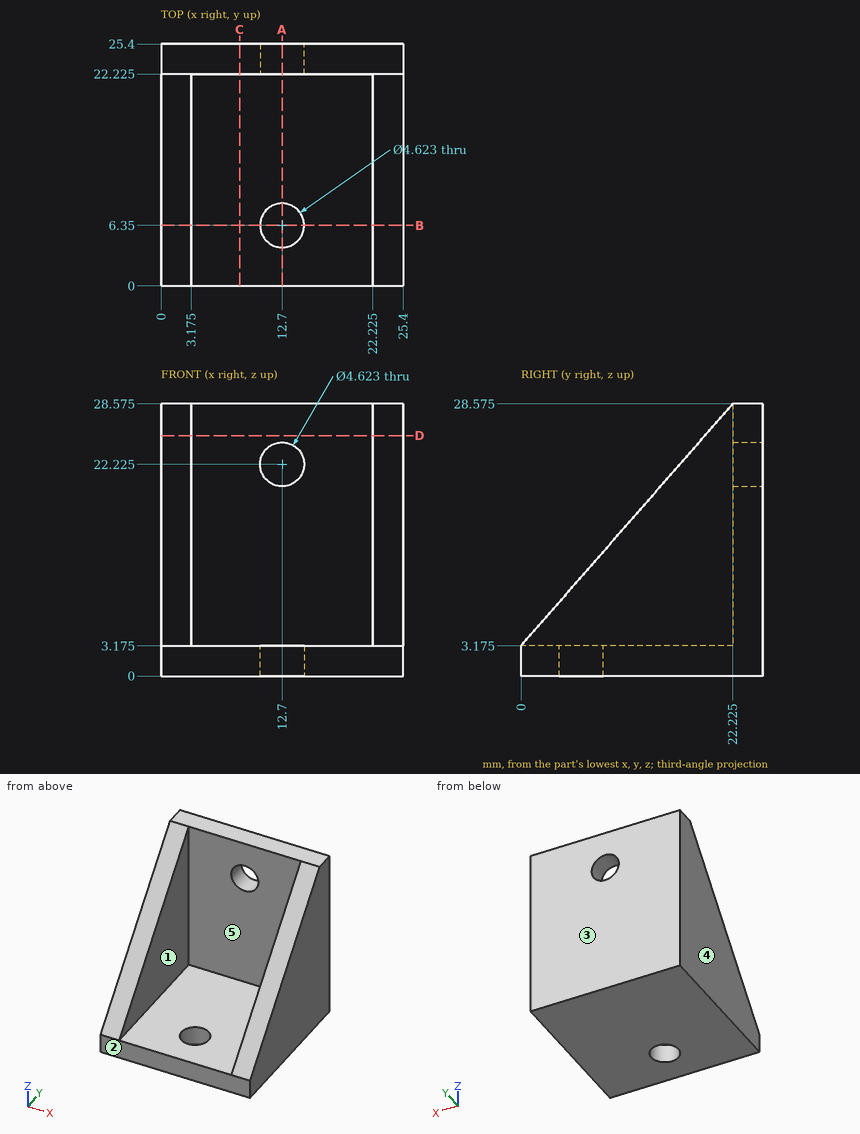
Source: three-view drawing plus pictorial views. Frame: mm from the lowest corner of the part. A direction names the side the tool comes from. Round coordinates to 2 decimals unless told otherwise and drop trailing zeros. Loops run counter-clockwise (first coordinate to the right, second up) from the corner with the lowest first, then second, coordinate; pieces in that order, holes last.
1. Section query A-A on x = 12.7. Output: boundary loops of the cut face in (y, z) (1 decimal).
2. Section query B-B on y = 6.35. Output: boundary loops of the cut face in (x, z) (1 decimal), and give its area (3 significant figures).
3. Section query D-D on z = 25.25. Output: boundary loops of the cut face in (x, y) (1 decimal).
4. Ray query, L1, parallel to X at y = 16.5, z = 11.5 (3 decimals); L2, parallel to Y at x = 12.7, z = 2.4; L3, parallel to Z at x = 12.7, y = 22.9 (1 decimal). Return the intervals inside material, ascending.
5. Contact query for flat-ended pins moving along their axis: pin 1 (10 mm diameter, centred on x = 12, y = 16.5, fed in from +Z) (3 decimals); pin 2 (3.5 mm diameter, centred on x = 12.7, y = 6.35, fed in from -Z); pin 3 (3 mm diameter, centred on x = 11.5, z = 13.5, fed in from -Y) (3 decimals). Output: stop coordinate, or through.
6. Section query C-C on x = 8.25. Output: boundary loops of the cut face in (y, z) (3 decimals).
7. Mould query, pull axis X, two halves, no side actions, for the marked faces 3, 4 and 5. Classes: released by +X, released by -X, zero draft, split by the parting line, or undercut.
8. Access query for the marked faces 1 and 2. Directions: +Z, -Z, +X, -X, +Y, -Y. A direction counts if a zero-diameter tool reaches every point of the face in a straight line with its end or side. Return the directions, or none.
Answers below:
1. outline: (0, 0) - (4, 0) - (4, 3.2) - (0, 3.2) - close; (8.7, 0) - (25.4, 0) - (25.4, 19.9) - (22.2, 19.9) - (22.2, 3.2) - (8.7, 3.2) - close; (22.2, 24.5) - (25.4, 24.5) - (25.4, 28.6) - (22.2, 28.6) - close
2. outline: (0, 0) - (10.4, 0) - (10.4, 3.2) - (3.2, 3.2) - (3.2, 10.4) - (0, 10.4) - close; (15, 0) - (25.4, 0) - (25.4, 10.4) - (22.2, 10.4) - (22.2, 3.2) - (15, 3.2) - close
2. area: 112 mm2
3. outline: (0, 19.3) - (3.2, 19.3) - (3.2, 22.2) - (22.2, 22.2) - (22.2, 19.3) - (25.4, 19.3) - (25.4, 25.4) - (0, 25.4) - close
4. L1: x = 0 to 3.175, 22.225 to 25.4
4. L2: y = 0 to 4.04, 8.66 to 25.4
4. L3: z = 0 to 19.9, 24.5 to 28.6
5. pin 1: stops at z = 3.175
5. pin 2: passes through
5. pin 3: stops at y = 22.225
6. outline: (0, 0) - (25.4, 0) - (25.4, 28.575) - (22.225, 28.575) - (22.225, 3.175) - (0, 3.175) - close
7. face 3: zero draft
7. face 4: released by -X
7. face 5: undercut
8. face 1: +Z, -Y
8. face 2: +Z, -Z, +X, -X, -Y
